Geometry check sheet. Reference: the model listing, model coordinates, mm. Give positions to 0.01 mm unless a question says otherwise; leave off trailing zeros. Order: outer loops, then holes, each group sorted by start corner. A loop starts at its lowest first (then second) coordinate and runs counter-clockwise, first axis right, second up.
Solid Edge part; units mm, degrees
sketch "Sketch1" plane through (0, 0, 0) normal (0, -1, 0) x (1, 0, 0)
  line L0 (75, -42) -> (75, 42)
  line L1 (75, 42) -> (-75, 42)
  line L2 (-75, 42) -> (-75, -42)
  line L3 (-75, -42) -> (75, -42)
extrude "Protrusion1" add sketch "Sketch1" along normal blind 2
sketch "Sketch2" plane through (0, 0, 0) normal (0, -1, 0) x (1, 0, 0)
  line L0 (-55, 38) -> (-55, 40)
  line L1 (-55, 40) -> (-65, 40)
  line L2 (-65, 40) -> (-65, 38)
  line L3 (-65, 38) -> (-55, 38)
  line L4 (-25, 40) -> (-35, 40)
  line L5 (-35, 40) -> (-35, 38)
  line L6 (-35, 38) -> (-25, 38)
  line L7 (-25, 38) -> (-25, 40)
  line L8 (-5, 38) -> (5, 38)
  line L9 (5, 38) -> (5, 40)
  line L10 (5, 40) -> (-5, 40)
  line L11 (-5, 40) -> (-5, 38)
  line L12 (25, 38) -> (35, 38)
  line L13 (35, 38) -> (35, 40)
  line L14 (35, 40) -> (25, 40)
  line L15 (25, 40) -> (25, 38)
  line L16 (55, 38) -> (65, 38)
  line L17 (65, 38) -> (65, 40)
  line L18 (65, 40) -> (55, 40)
  line L19 (55, 40) -> (55, 38)
  line L20 (65, -40) -> (65, -38)
  line L21 (65, -38) -> (55, -38)
  line L22 (55, -38) -> (55, -40)
  line L23 (55, -40) -> (65, -40)
  line L24 (25, -40) -> (35, -40)
  line L25 (35, -40) -> (35, -38)
  line L26 (35, -38) -> (25, -38)
  line L27 (25, -38) -> (25, -40)
  line L28 (5, -38) -> (-5, -38)
  line L29 (-5, -38) -> (-5, -40)
  line L30 (-5, -40) -> (5, -40)
  line L31 (5, -40) -> (5, -38)
  line L32 (-25, -38) -> (-35, -38)
  line L33 (-35, -38) -> (-35, -40)
  line L34 (-35, -40) -> (-25, -40)
  line L35 (-25, -40) -> (-25, -38)
  line L36 (-55, -40) -> (-55, -38)
  line L37 (-55, -38) -> (-65, -38)
  line L38 (-65, -38) -> (-65, -40)
  line L39 (-65, -40) -> (-55, -40)
  line L40 (-73, -42) -> (-73, -25)
  line L41 (-73, -25) -> (-75, -25)
  line L42 (-75, -25) -> (-75, -42)
  line L43 (-75, -42) -> (-73, -42)
  line L44 (-73, -15) -> (-73, -5)
  line L45 (-73, -5) -> (-75, -5)
  line L46 (-75, -5) -> (-75, -15)
  line L47 (-75, -15) -> (-73, -15)
  line L48 (-73, 5) -> (-73, 15)
  line L49 (-73, 15) -> (-75, 15)
  line L50 (-75, 15) -> (-75, 5)
  line L51 (-75, 5) -> (-73, 5)
  line L52 (-73, 25) -> (-73, 42)
  line L53 (-73, 42) -> (-75, 42)
  line L54 (-75, 42) -> (-75, 25)
  line L55 (-75, 25) -> (-73, 25)
  line L56 (75, 25) -> (75, 42)
  line L57 (75, 42) -> (73, 42)
  line L58 (73, 42) -> (73, 25)
  line L59 (73, 25) -> (75, 25)
  line L60 (73, 15) -> (73, 5)
  line L61 (73, 5) -> (75, 5)
  line L62 (75, 5) -> (75, 15)
  line L63 (75, 15) -> (73, 15)
  line L64 (73, -5) -> (73, -15)
  line L65 (73, -15) -> (75, -15)
  line L66 (75, -15) -> (75, -5)
  line L67 (75, -5) -> (73, -5)
  line L68 (73, -25) -> (73, -42)
  line L69 (73, -42) -> (75, -42)
  line L70 (75, -42) -> (75, -25)
  line L71 (75, -25) -> (73, -25)
extrude "ExtrudedCutout_1" cut sketch "Sketch2" along normal blind 2
properties material "Acrylic, high impact grade"
Item 1: Sectioned sample at C-C (y = -0.9). Give the number of separate pieces and of enclosed holes in the cut face, and give its area (3 significant figures).
Reported:
separate pieces: 1
enclosed holes: 10
area: 12,200 mm2
Item 2: Sectioned sample at A-A (x = -58). Enter the section's corners in (y, z).
Reported:
outline: (-2, -42) - (0, -42) - (0, -40) - (-2, -40) - close; (-2, -38) - (0, -38) - (0, 38) - (-2, 38) - close; (-2, 40) - (0, 40) - (0, 42) - (-2, 42) - close
Item 3: Gauge pin test, flat ends, axial feed: pin 1 (10 mm diameter, centred on x = -44, z = 23.5, fed in from +Y); pin 2 (1 mm diameter, centred on y = -1.5, z = 30.5, fed in from +X); pin 3 (0.6 mm diameter, centred on y = -1.5, z = -39.5, fed in from -X); pin 4 (0.6 mm diameter, centred on x = 74.5, y = -1, fed in from +Z). Record the tip position at first contact, or that the pin passes through.
Reported:
pin 1: stops at y = 0
pin 2: stops at x = 73
pin 3: stops at x = -73
pin 4: stops at z = 25
Item 4: Sectioned sample at B-B (z = -30.5). Enter the section's corners in (x, y), and give its area (3 significant figures).
Reported:
outline: (-73, -2) - (73, -2) - (73, 0) - (-73, 0) - close
area: 292 mm2
Item 5: Scan lines: L1, parallel to Z at x = -31, y = -1.8; L2, parallel to X at y = -1.5, z = 36. Record each from-to range of solid material in increasing order.
Reported:
L1: z = -42 to -40, -38 to 38, 40 to 42
L2: x = -73 to 73
